For this review, use the dimensioned drawing (mm, ordinates from the lowest corner) and the shaded views. A direction names the side the tool comes from. Give positions to 0.01 mm unless a question says otherwise; leave off trailing zeros. Write each loop counter-clockwise with the first axis right and the second up, starting at its lowest first coordinate (ties: lowest second). Pieces come first, ordered by that corner, then holes.
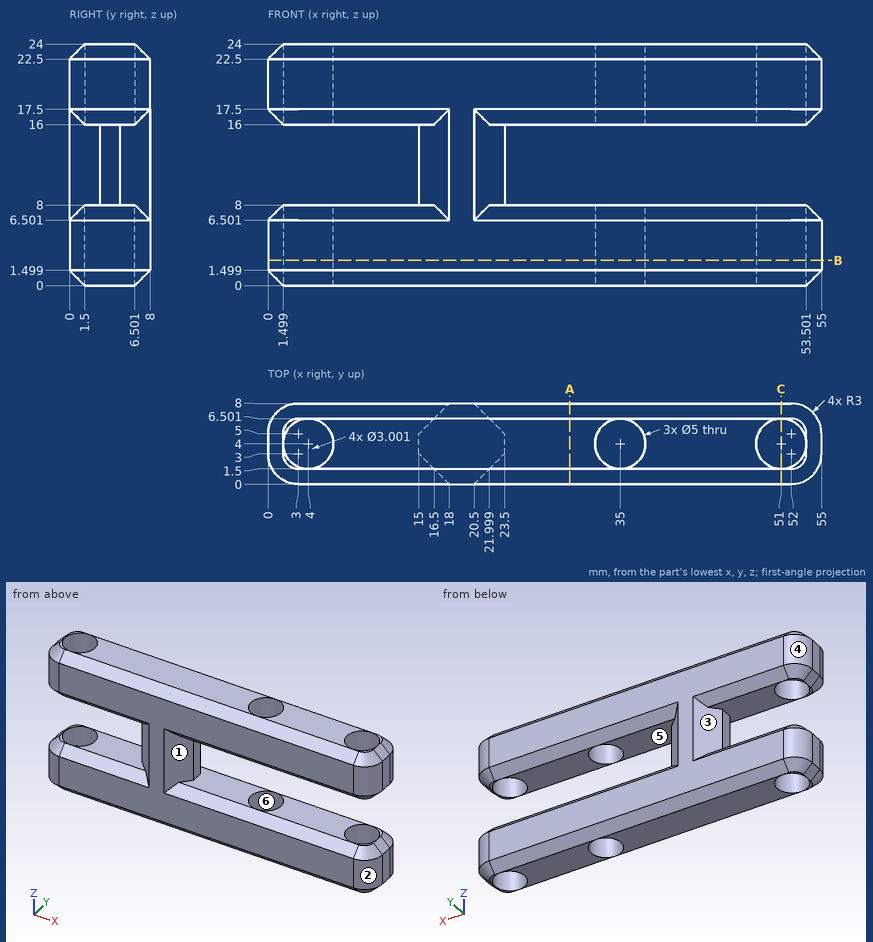
(1) Tool access review of the marked faces 1, 2 and 3: name each direction out of +Z, -Z, +X, -X, +Y, -Y from which nothing blocks a thin tool from reaching the whole face with its end or side.
(2) The part is to be moulded in two halves that separate along X. For the marked faces 4, 5 and 6, say which applies: +X half, -X half, draft (parallel to the pull), parting line (faces both ways), or undercut.
(3) We need section A-A (x = 30). Write out the cut boundary in (y, z), and give its area (3 significant figures).
(4) Clearance check with flat-ended pins moving along their axes: pin 1 Ø8 at (x, z) = (23, 19.5) entering from -Y; pin 2 Ø1 at (y, z) = (4, 11) entering from -X; pin 3 Ø1.5 at (y, z) = (6.5, 6.5) entering from -X (1 decimal); pin 4 Ø1 at (y, z) = (4, 12) entering from +X. State where each tip first meets the part, or that it passes through.
(5) For L1, parallel to X at y = 3.75, z = 1.75; L2, parallel to Z at x = 29, y = 2; L3, parallel to Y at x = 4, z = 2, list the stretches that pass through material, from the lowest coordinate up.
(6) We need section B-B (z = 2.5). Write out the cut boundary in (x, y).
(7) We need section C-C (x = 51). Count the separate pieces of the cut face and the enclosed holes in it.
The answers:
1. face 1: +X, -Y
1. face 2: +Z, -Z, +X, -Y
1. face 3: -X, +Y
2. face 4: -X half
2. face 5: draft
2. face 6: undercut
3. outline: (0, 1.5) - (1.5, 0) - (6.5, 0) - (8, 1.5) - (8, 6.5) - (6.5, 8) - (1.5, 8) - (0, 6.5) - close; (0, 17.5) - (1.5, 16) - (6.5, 16) - (8, 17.5) - (8, 22.5) - (6.5, 24) - (1.5, 24) - (0, 22.5) - close
3. area: 119 mm2
4. pin 1: stops at y = 0
4. pin 2: stops at x = 15
4. pin 3: stops at x = 0.1
4. pin 4: stops at x = 23.5
5. L1: x = 0 to 1.51, 6.49 to 32.51, 37.49 to 48.51, 53.49 to 55
5. L2: z = 0 to 8, 16 to 24
5. L3: y = 0 to 1.5, 6.5 to 8
6. outline: (0, 3) arc R3 ccw to (3, 0) - (52, 0) arc R3 ccw to (55, 3) - (55, 5) arc R3 ccw to (52, 8) - (3, 8) arc R3 ccw to (0, 5) - close; hole circle Ø5 at (4, 4); hole circle Ø5 at (35, 4); hole circle Ø5 at (51, 4)
7. separate pieces: 4
7. enclosed holes: 0
